from build123d import *

# Parameters (mm, degrees)
SKETCH4_W           = 80
SKETCH4_H           = 80
BOSS_EXTRUDE1_DEPTH = 40
SKETCH5_R           = 20
BOSS_EXTRUDE2_DEPTH = 10
CHAMFER1_SIZE       = 10


with BuildPart() as part:
    # Sketch4 → Boss-Extrude1 (new body)
    with BuildSketch(Plane(origin=(0, 0, 0), x_dir=(1, 0, 0), z_dir=(0, 1, 0))):
        Rectangle(SKETCH4_W, SKETCH4_H)
    extrude(amount=BOSS_EXTRUDE1_DEPTH)

    # Sketch5 → Boss-Extrude2 (add)
    with BuildSketch(Plane(origin=(0, 40, 0), x_dir=(1, 0, 0), z_dir=(0, 1, 0))):
        with Locations(Location((0, 0, 0), (0, 0, 270))):
            Circle(SKETCH5_R)
    extrude(amount=BOSS_EXTRUDE2_DEPTH)

    # Chamfer1
    chamfer1_edges = [part.edges().sort_by_distance(p)[0] for p in [
        (40, 40, 0),
        (0, 40, -40),
        (-40, 40, 0),
        (0, 40, 40),
    ]]
    chamfer(chamfer1_edges, length=CHAMFER1_SIZE)


solid = part.part
Design review of the part built by this model. Coordinates are the model's own, in mm. A direction names the side the tool comes from. Coordinates: 2 decimals unless noted, no trailing zeros. Order: outer loops, then holes, each group sorted by start corner. A loop starts at its lowest first (then second) coordinate and runs counter-clockwise, first axis right, second up. Notation, with made-up numbers: (52, 70.5) -> (108, 70.5) arc R22 ccw to (108, 102.5) -> close; hole circle Ø4 at (40, 77.25). An arc over 180 degrees is marked (long way). One line per item, written item: value.
1) We need section D-D, the plane x = 33. Give the boundary of the cut face in (y, z), then the cut area to 3 significant figures.
Output values:
outline: (0, -40) -> (30, -40) -> (37, -33) -> (37, 33) -> (30, 40) -> (0, 40) -> close
area: 2,910 mm2
2) We need section A-A, the plane x = 0. Give the boundary of the cut face in (y, z).
Output values:
outline: (0, -40) -> (30, -40) -> (40, -30) -> (40, -20) -> (50, -20) -> (50, 20) -> (40, 20) -> (40, 30) -> (30, 40) -> (0, 40) -> close
3) Clearance check with flat-ended pins moving along their axes: P1, Ø1, axis at y = 31, z = 0, coming from the +X side; P2, Ø8, axis at x = -27, z = -7.5, coming from the +Y side; P3, Ø5, axis at y = 35, z = 31.5, coming from the +X side. State where each tip first meets the part, or that it passes through.
Output values:
P1: stops at x = 39.5
P2: stops at y = 40
P3: stops at x = 37.5
4) We need section B-B, the plane z = 0. Give the boundary of the cut face in (x, y), then the cut area to 3 significant figures.
Output values:
outline: (-40, 0) -> (40, 0) -> (40, 30) -> (30, 40) -> (20, 40) -> (20, 50) -> (-20, 50) -> (-20, 40) -> (-30, 40) -> (-40, 30) -> close
area: 3,500 mm2
5) To check wall thickness, follow probe 1 along Y at (x, z) = (21, 19); probe 2 along Y at (x, z) = (-31, 20); probe 3 along Z at (x, y) = (3, 38.5). State the ranges of each line that lie inside material, in increasing order. Write a range as [from, to].
Output values:
probe 1: y = [0, 40]
probe 2: y = [0, 39]
probe 3: z = [-31.5, 31.5]
6) We need section C-C, the plane z = -24. Give the boundary of the cut face in (x, y).
Output values:
outline: (-40, 0) -> (40, 0) -> (40, 30) -> (30, 40) -> (-30, 40) -> (-40, 30) -> close
7) Machinability: for faces 1 (the face through (-40, 15, 1)), 2 (the face through (-19.524, 44.93, -4.336)), which of the approach directions +Z, -Z, +X, -X, +Y, -Y give a long, thin tool a straight path to every point of the face, cutting with its end or side? Answer none if there is none.
Output values:
face 1: +Z, -Z, -X, +Y, -Y
face 2: +Y
